Autodesk Inventor part; units mm, degrees
ref_plane "YZ Plane" through (0, 0, 0) normal (1, 0, 0) x (0, 1, 0)
ref_plane "XZ Plane" through (0, 0, 0) normal (0, 1, 0) x (-1, 0, 0)
ref_plane "XY Plane" through (0, 0, 0) normal (0, 0, 1) x (1, 0, 0)
sketch "Sketch1" plane through (0, 0, 0) normal (0, 1, 0) x (-1, 0, 0)
  line L0 (0, 0) -> (40.2, 0)
  line L1 (40.2, 0) -> (40.2, 60.3)
  line L2 (40.2, 60.3) -> (0, 60.3)
  line L3 (0, 60.3) -> (0, 0)
  dimension "d0" = 60.3
  dimension "d1" = 40.2
extrude "Extrusion1" add sketch "Sketch1" along normal blind 24
sketch "Sketch2" plane through (-40.2, 0, 60.3) normal (0, 0, 1) x (1, 0, 0)
  line L0 (0, 0) -> (40.2, 0)
  line L1 (40.2, 0) -> (40.2, 24)
  line L2 (0, 24) -> (40.2, 24)
  line L3 (0, 0) -> (0, 24)
  line L4 (40.2, 24) -> (28.2, 24)
  line L5 (28.2, 24) -> (28.2, 15.2)
  line L6 (28.2, 15.2) -> (40.2, 15.2)
  line L7 (40.2, 15.2) -> (40.2, 24)
  point P0 (40.2, 0)
  point P1 (28.2, 24)
  dimension "d4" = 12
  dimension "d5" = 8.8
extrude "Extrusion2" cut sketch "Sketch2" against normal through all contours L6 L5 L2 L1
sketch "Sketch3" plane through (0, 0, 60.3) normal (1, 0, 0) x (0, 0, -1)
  line L0 (60.3, 15.2) -> (0, 15.2)
  line L1 (0, 0) -> (0, 15.2)
  line L2 (0, 0) -> (60.3, 0)
  line L3 (60.3, 0) -> (60.3, 15.2)
  line L4 (60.3, 15.2) -> (35.3, 15.2)
  line L5 (35.3, 15.2) -> (35.3, 7.8)
  line L6 (35.3, 7.8) -> (60.3, 7.8)
  line L7 (60.3, 7.8) -> (60.3, 15.2)
  dimension "d8" = 25
  dimension "d9" = 7.4
extrude "Extrusion3" cut sketch "Sketch3" against normal up to surface (12 mm away) contours L3 L6 L5 L0
properties part number "New Board"
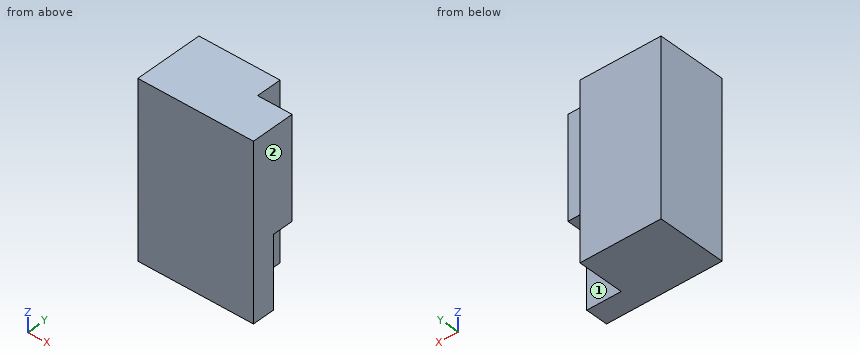
Input: part model. Units: mm. Frame: model coordinates. Face numbers are marked on the shaded views. A direction names the side the tool comes from. Coordinates: 2 decimals unless noted, no trailing zeros. Write each loop counter-clockwise with the first axis right and the second up, starting at its lowest first coordinate (ties: lowest second). Pieces come first, ordered by that corner, then holes.
1) Material intervals for line 1 along X through (y, z) = (18.75, 9); line 2 along Y through (x, z) = (-2, 18.5); line 3 along Y through (x, z) = (-10, 31.5), sorted ascending.
2) Section B-B on z = 47. Output: boundary loops of the cut face in (x, y), and give its area (3 significant figures).
3) Pin query (flat end, axial travel): pin 1 Ø12 at (x, z) = (-5.5, 19.5) entering from +Y; pin 2 Ø8 at (y, z) = (20, 44.5) entering from +X; pin 3 Ø6 at (x, y) = (-8, 12) entering from -Z; pin 4 Ø1 at (y, z) = (5.5, 11) entering from +X. Return the tip coordinate at first contact, or that it passes through.
4) Set-up query: the marked faces 1 and 2. Return all of +Z, -Z, +X, -X, +Y, -Y with unobstructed straight access to the full face (end or side cutting, diameter ignored); none if empty.
5) Section C-C on y = 20.5. Output: boundary loops of the cut face in (x, z), and give its area (3 significant figures).
6) Section A-A on y = 9.75. Output: boundary loops of the cut face in (x, z).
Check result:
1. line 1: x = -40.2 to -12
1. line 2: y = 0 to 7.8
1. line 3: y = 0 to 15.2
2. outline: (-40.2, 0) - (0, 0) - (0, 15.2) - (-12, 15.2) - (-12, 24) - (-40.2, 24) - close
2. area: 859 mm2
3. pin 1: stops at y = 15.2
3. pin 2: stops at x = -12
3. pin 3: stops at z = 25
3. pin 4: stops at x = 0
4. face 1: -Z, +X, +Y
4. face 2: +Z, -Z, +X, +Y, -Y
5. outline: (-40.2, 0) - (-12, 0) - (-12, 60.3) - (-40.2, 60.3) - close
5. area: 1,700 mm2
6. outline: (-40.2, 0) - (-12, 0) - (-12, 25) - (0, 25) - (0, 60.3) - (-40.2, 60.3) - close
